Autodesk Inventor part; units mm, degrees
ref_plane "YZ Plane" through (0, 0, 0) normal (1, 0, 0) x (0, 1, 0)
ref_plane "XZ Plane" through (0, 0, 0) normal (0, 1, 0) x (-1, 0, 0)
ref_plane "XY Plane" through (0, 0, 0) normal (0, 0, 1) x (1, 0, 0)
sketch "Sketch1" plane through (0, 0, 0) normal (0, 0, 1) x (1, 0, 0)
  line L0 (-10, -12.5) -> (10, -12.5) construction
  line L1 (10, -12.5) -> (10, 12.5) construction
  line L2 (10, 12.5) -> (-10, 12.5) construction
  line L3 (-10, 12.5) -> (-10, -12.5) construction
  line L4 (-10, -12.5) -> (10, 12.5) construction
  line L5 (10, -12.5) -> (-10, 12.5) construction
  circle A0 centre (-10, 12.5) radius 1.925
  circle A1 centre (10, 12.5) radius 1.925
  circle A2 centre (10, -12.5) radius 1.925
  circle A3 centre (-10, -12.5) radius 1.925
  arc A4 (-7.1685, 17.7046) -> (-15.1908, 9.6432) centre (-10, 12.5) ccw
  arc A5 (15.1908, 9.6432) -> (7.1685, 17.7046) centre (10, 12.5) ccw
  arc A6 (7.1685, -17.7046) -> (15.1908, -9.6432) centre (10, -12.5) ccw
  arc A7 (-15.1908, -9.6432) -> (-7.1685, -17.7046) centre (-10, -12.5) ccw
  arc A8 (-7.1685, 17.7046) -> (7.1685, 17.7046) centre (0, 30.8808) ccw
  arc A9 (7.1685, -17.7046) -> (-7.1685, -17.7046) centre (0, -30.8808) ccw
  arc A10 (15.1908, 9.6432) -> (15.1908, -9.6432) centre (32.7125, 0) ccw
  arc A11 (-15.1908, -9.6432) -> (-15.1908, 9.6432) centre (-32.7125, 0) ccw
  point P0 (0, 0)
  dimension "d0" = 25
  dimension "d1" = 20
  dimension "d2" = 3.85
  dimension "d3" = 4
  dimension "d4" = 15
  dimension "d5" = 20
extrude "Extrusion1" add sketch "Sketch1" along normal blind 5
sketch "Sketch2" plane through (0, 0, 5) normal (0, 0, 1) x (1, 0, 0)
  circle A0 centre (0, 0) radius 4 construction
  line L0 (-1, -4.35) -> (1, -4.35)
  line L1 (1, -4.35) -> (5.0946, -1)
  line L2 (5.0946, -1) -> (12, -1)
  line L3 (-1, -4.35) -> (-5.0946, -1)
  line L4 (-5.0946, -1) -> (-12, -1)
  line L5 (0, 0) -> (0, -4.35) construction
  line L6 (-12, -1) -> (-12, -4)
  line L7 (-12, -4) -> (-4.899, -4)
  line L8 (12, -1) -> (12, -4)
  line L9 (12, -4) -> (4.899, -4)
  arc A1 (-4.899, -4) -> (4.899, -4) centre (0, -1.5) ccw
  dimension "d8" = 8
  dimension "d9" = 1
  dimension "d10" = 3
  dimension "d11" = 24
  dimension "d12" = 2
  dimension "d13" = 3.35
  dimension "d14" = 5.5
  dimension "d15" = 2.5
extrude "Extrusion2" add sketch "Sketch2" along normal blind 15
sketch "Sketch3" plane through (4.899, -4, 5) normal (0, -1, 0) x (1, 0, 0)
  line L0 (7.101, 0) -> (0, 0)
  line L1 (7.101, 0) -> (7.101, 15)
  line L2 (0, 0) -> (0, 15)
  circle A0 centre (3.5505, 7.5) radius 1.6
  circle A1 centre (-13.3485, 7.5) radius 1.6
  line L3 (3.5505, 0) -> (3.5505, 7.5) construction
  line L4 (3.5505, 7.5) -> (7.101, 7.5) construction
  line L5 (-16.899, 7.5) -> (-13.3485, 7.5) construction
  line L6 (-13.3485, 7.5) -> (-13.3485, 0) construction
  line L7 (-16.899, 0) -> (-16.899, 15)
  point P0 (-4.899, -5)
  dimension "d18" = 3.2
extrude "Extrusion3" cut sketch "Sketch3" against normal blind 15
sketch "Sketch4" plane through (0, 0, 5) normal (0, 0, 1) x (1, 0, 0)
  line L0 (1, -4.35) -> (5.0946, -1)
  line L1 (-5.0946, -1) -> (-1, -4.35)
  line L2 (-1, -4.35) -> (1, -4.35)
  line L3 (-5.0946, -1) -> (-1, -4.35)
  line L4 (-1, -4.35) -> (1, -4.35)
  line L5 (1, -4.35) -> (5.0946, -1)
  line L6 (5.0946, 21.1209) -> (-5.0946, 21.1209)
  line L7 (-5.0946, 21.1209) -> (-5.0946, -1)
  line L8 (5.0946, -1) -> (5.0946, 21.1209)
  point P0 (0, 0)
extrude "Extrusion4" cut sketch "Sketch4" against normal blind 10
sketch "Sketch5" plane through (-12, -1, 20) normal (0, 1, 0) x (1, 0, 0)
  line L0 (0, 15) -> (6.9054, 15)
  line L1 (-11.2791, 15) -> (33.3469, 15)
  line L2 (33.3469, 15) -> (33.3469, 24.5778)
  line L3 (33.3469, 24.5778) -> (-11.2791, 24.5778)
  line L4 (-11.2791, 24.5778) -> (-11.2791, 15)
  point P0 (12, 20)
extrude "Extrusion5" cut sketch "Sketch5" against normal blind 25.875 and the other way blind 28.8125
sketch "Sketch6" plane through (-5.0946, -1, 5) normal (0, 0, -1) x (-1, 0, 0)
  line L0 (-10.1893, 0) -> (-6.0946, -3.35)
  line L1 (-10.1893, 0) -> (-17.0946, 0)
  line L2 (-17.0946, 0) -> (-17.0946, -3)
  line L3 (-17.0946, -3) -> (-9.9936, -3)
  arc A0 (-9.9936, -3) -> (-0.1957, -3) centre (-5.0946, -0.5) ccw
  line L4 (-0.1957, -3) -> (6.9054, -3)
  line L5 (6.9054, -3) -> (6.9054, 0)
  line L6 (6.9054, 0) -> (0, 0)
  line L7 (-4.0946, -3.35) -> (0, 0)
  line L8 (-6.0946, -3.35) -> (-4.0946, -3.35)
  line L9 (-17.0946, 0) -> (-10.1893, 0)
  line L10 (-6.0946, -3.35) -> (-10.1893, 0)
  line L11 (-6.0946, -3.35) -> (-4.0946, -3.35)
  line L12 (-4.0946, -3.35) -> (0, 0)
  line L13 (0, 0) -> (6.9054, 0)
  line L14 (6.9054, 0) -> (6.9054, -12)
  line L15 (6.9054, -12) -> (-17.0946, -12)
  line L16 (-17.0946, -12) -> (-17.0946, 0)
  point P0 (-5.0946, 1)
  dimension "d36" = 12
extrude "Extrusion6" add sketch "Sketch6" against normal blind 2 contours L3 A0 L4 L14 L15 L16
chamfer "Chamfer2" distance 1 angle 45 3 edges at (-8.4495, -4, 7) (0, -7, 7) (8.4495, -4, 7)
fillet "Fillet6" radius 0.75 21 edges at (12, -4, 14) (12, -1, 12.5) (-12, -4, 14) (-12, -1, 12.5) (-4.899, -4, 14) (4.899, -4, 14) (5.0946, -1, 12.5) (1, -4.35, 12.5) (-1, -4.35, 12.5) (-5.0946, -1, 12.5) (6.8495, -4, 12.5) (6.8495, -1, 12.5) (-10.0495, -4, 12.5) (-10.0495, -1, 12.5) (-12, -4.5, 7.5) (-12, -9, 7) (12, -4.5, 7.5) (12, -9, 7) (0, -13, 7) (12, -13, 6) (-12, -13, 6)
properties part number "rodClamp"
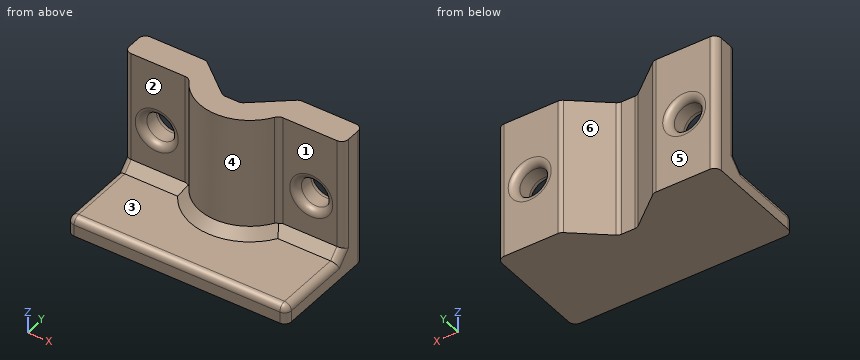
Work out the finished part from the listing and answer in its coordinate system (mm). Face numbers are marked on the shaded views. A direction names the side the tool comes from. Coordinates: 2 decimals unless noted, no trailing zeros. Order: outer loops, then holes, each group sorted by start corner. A loop starts at its lowest first (then second) coordinate and runs counter-clockwise, first axis right, second up. Notation, with made-up numbers: M 74,77.5 L 83,77.5 A11 ccw 83,89.5 Z; hole C -13.75,57 d5. An arc over 180 degrees is marked long. Use CSV: the item, a comma, the result in double quotes.
1) Determine the mould class of the marked faces 4, 5 and 6 for opening direction X: released by +X, released by -X, zero draft, split by the parting line, or undercut.
Worked out:
face 4,"split by the parting line"
face 5,"zero draft"
face 6,"undercut"
2) For the marked faces 1, 2 and 3, determine the directions among +Z, -Z, +X, -X, +Y, -Y from which every point of the face is accessible in a straight line to the end or side of a thin tool.
Worked out:
face 1,"+Z, +X, -Y"
face 2,"+Z, -X, -Y"
face 3,"+Z, -Y"
3) Consider line 1 (Y direction, x = 10, z = 16); line 2 (Z direction, x = -4.75, y = -10.75); line 3 (X direction, y = -1.75, z = 19). Determine where each line is inside the solid, lowest interval first. Write a range as [from, to].
Worked out:
line 1,"y = [-4, -1]"
line 2,"z = [5, 7]"
line 3,"x = [-12, -4.18], [4.18, 12]"
4) Section B-B on z = 12.5 is taken. Count the separate pieces of the cut face and the enclosed holes in it, plus the area to 3 significant figures.
Worked out:
separate pieces,"3"
enclosed holes,"0"
area,"52.0 mm^2"
5) Flat-ended cylindrical pins translate along their axes: pin 1 Ø4 at (x, z) = (-0.5, 16.5) entering from +Y; pin 2 Ø8 at (x, z) = (3.5, 9) entering from -Y; pin 3 Ø4 at (x, z) = (-8.45, 12.5) entering from +Y; pin 4 Ø2 at (x, z) = (4.5, 12.5) entering from -Y. Find the tip coordinate at first contact, or state that the pin passes through.
Worked out:
pin 1,"stops at y = -3.12"
pin 2,"stops at y = -13"
pin 3,"stops at y = -1.09"
pin 4,"stops at y = -5.74"
6) Section C-C on y = -8.25 is taken. Write down the section's boundary in (x, z), plus the area to 3 significant figures.
Worked out:
outline,"M -12,5 L 12,5 L 12,6.25 A0.75 ccw 11.25,7 L -11.25,7 A0.75 ccw -12,6.25 Z"
area,"47.8 mm^2"
7) Section A-A on y = -3 is taken. Write down the section's boundary in (x, z).
Worked out:
outline,"M -12,5 L -2.65,5 L -2.65,20 L -12,20 Z; M 2.65,5 L 12,5 L 12,20 L 2.65,20 Z; hole C -8.45,12.5 d3.2; hole C 8.45,12.5 d3.2"
8) Section D-D on z = 18.5 is taken. Write down the section's boundary in (x, y), plus the area to 3 significant figures.
Worked out:
outline,"M -12,-3.25 A0.75 ccw -11.25,-4 L -5.34,-4 A0.75 cw -4.7,-4.36 A5.5 ccw 4.7,-4.36 A0.75 cw 5.34,-4 L 11.25,-4 A0.75 ccw 12,-3.25 L 12,-1.75 A0.75 ccw 11.25,-1 L 5.36,-1 A0.75 ccw 4.89,-1.17 L 1.21,-4.18 A0.75 cw 0.73,-4.35 L -0.73,-4.35 A0.75 cw -1.21,-4.18 L -4.89,-1.17 A0.75 ccw -5.36,-1 L -11.25,-1 A0.75 ccw -12,-1.75 Z"
area,"72.2 mm^2"
